Geometry: final body of the model. Coordinates: model frame, mm. Face numbers are marked on the shaded views. A direction names the side the tool comes from. Round coordinates to 2 decimals unless told otherwise and drop trailing zeros. Order: outer loops, then holes, each group sorted by start corner. A loop starts at its lowest first (then second) coordinate and runs counter-clockwise, first axis right, second up. Notation, with made-up numbers: (57, 13) -> (87, 13) arc R24 ccw to (87, 41) -> close; hole circle Ø7 at (23, -29). An arc over 180 degrees is marked (long way). Put each result on its own line as item: value.
```python
from build123d import *

# Parameters (mm, degrees)
SKETCH1_W           = 128.5875
SKETCH1_H           = 144.4625
BOSS_EXTRUDE1_DEPTH = 61.07176
SHELL1_T            = 6.35
SKETCH2_R           = 8.73125
SKETCH2_R_2         = 19.84375
SKETCH2_W           = 45.72
SKETCH2_H           = 63.1825
SKETCH2_W_2         = 69.215
SKETCH2_H_2         = 23.8125
CUT_EXTRUDE1_DEPTH  = 126.344509202
SKETCH3_W           = 31.75
SKETCH3_H           = 66.675
CUT_EXTRUDE2_DEPTH  = 6.35
SKETCH4_R           = 19.84375
SKETCH4_R_2         = 16.66875
BOSS_EXTRUDE2_DEPTH = 1.5875
SKETCH5_W           = 63.5
SKETCH5_H           = 12.7
CUT_EXTRUDE3_DEPTH  = 6.35
FILLET1_R           = 9.525
FILLET2_R           = 3.175


with BuildPart() as part:
    # Sketch1 → Boss-Extrude1 (new body)
    with BuildSketch(Plane.XY):
        Rectangle(SKETCH1_W, SKETCH1_H)
    extrude(amount=-BOSS_EXTRUDE1_DEPTH)

    # Shell1
    shell1_openings = [part.faces().sort_by_distance(p)[0] for p in [
        (0, 0, -61.07176),
    ]]
    offset(amount=SHELL1_T, openings=shell1_openings, kind=Kind.INTERSECTION)

    # Sketch2 → Cut-Extrude1 (cut, through all)
    with BuildSketch(Plane.XY.offset(6.35)):
        with Locations((-31.75, 50.8)):
            Circle(SKETCH2_R)
        with Locations((-31.75, 9.525)):
            Circle(SKETCH2_R_2)
        with Locations((26.19375, 25.4)):
            Rectangle(SKETCH2_W, SKETCH2_H)
        with Locations((11.90625, -41.275)):
            Rectangle(SKETCH2_W_2, SKETCH2_H_2)
    extrude(amount=-CUT_EXTRUDE1_DEPTH, mode=Mode.SUBTRACT)

    # Sketch3 → Cut-Extrude2 (cut)
    with BuildSketch(Plane(origin=(70.64375, 0, 0), x_dir=(0, 0, -1), z_dir=(1, 0, 0))):
        with Locations((31.39694, -13.43025)):
            Rectangle(SKETCH3_W, SKETCH3_H)
    extrude(amount=-CUT_EXTRUDE2_DEPTH, mode=Mode.SUBTRACT)

    # Sketch4 → Boss-Extrude2 (add)
    with BuildSketch(Plane.XY.offset(6.35)):
        with Locations((-31.75, 9.525)):
            Circle(SKETCH4_R)
        with Locations((-31.75, 9.525)):
            Circle(SKETCH4_R_2, mode=Mode.SUBTRACT)
    extrude(amount=-BOSS_EXTRUDE2_DEPTH)

    # Sketch5 → Cut-Extrude3 (cut)
    with BuildSketch(Plane(origin=(0, 78.58125, 0), x_dir=(1, 0, 0), z_dir=(0, 1, 0))):
        with Locations((0, 54.72176)):
            Rectangle(SKETCH5_W, SKETCH5_H)
    extrude(amount=-CUT_EXTRUDE3_DEPTH, mode=Mode.SUBTRACT)

    # Fillet1
    fillet1_edges = [part.edges().sort_by_distance(p)[0] for p in [
        (0, -78.58125, 6.35),
        (70.64375, 0, 6.35),
        (0, 78.58125, 6.35),
        (-70.64375, 0, 6.35),
        (-70.64375, -78.58125, -27.36088),
        (70.64375, -78.58125, -27.36088),
        (70.64375, 78.58125, -27.36088),
        (-70.64375, 78.58125, -27.36088),
    ]]
    fillet(fillet1_edges, radius=FILLET1_R)

    # Fillet2
    fillet2_edges = [part.edges().sort_by_distance(p)[0] for p in [
        (-64.29375, 0, 0),
        (-64.29375, -72.23125, -30.53588),
        (0, 72.23125, 0),
        (-64.29375, 72.23125, -30.53588),
        (64.29375, 72.23125, -30.53588),
        (64.29375, -72.23125, -30.53588),
        (0, -72.23125, 0),
        (64.29375, 0, 0),
    ]]
    fillet(fillet2_edges, radius=FILLET2_R)


solid = part.part
```
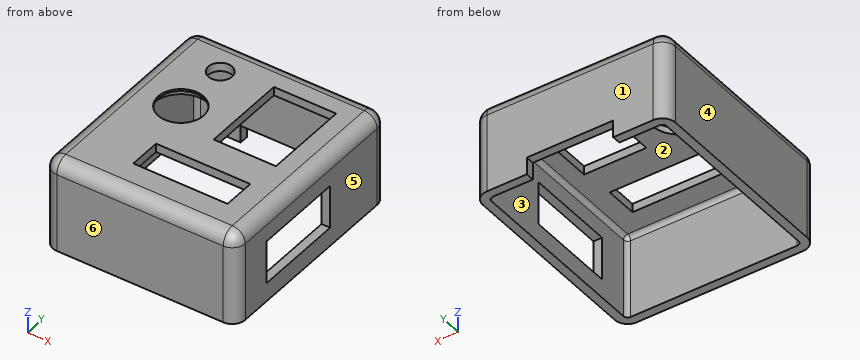
1. Draft query along X for the marked faces 3, 4, 5 and 6. Return one class per face: +X half, -X half, draft (parallel to the pull), parting line (faces both ways), or undercut.
Ans:
face 3: undercut
face 4: -X half
face 5: +X half
face 6: draft
2. Contact query for flat-ended pins moving along their axis: P1, Ø7, axis at x = 29, z = 4, coming from the +Y side; P2, Ø1.9, axis at y = 75, z = -55, coming from the -X side; P3, Ø5, axis at y = -46, z = 3.5, coming from the -X side. Output: stop coordinate, or through.
Ans:
P1: y = 77.84
P2: x = -69.23
P3: x = -69.68
3. Cut plane B-B on x = 53. Return loops of the section in (y, z) (3 decimals), and give its area (3 significant figures).
Ans:
outline: (-78.581, -61.072) -> (-72.231, -61.072) -> (-72.231, -3.175) arc R3.175 cw to (-69.056, 0) -> (69.056, 0) arc R3.175 cw to (72.231, -3.175) -> (72.231, -61.072) -> (78.581, -61.072) -> (78.581, -3.175) arc R9.525 ccw to (69.056, 6.35) -> (-69.056, 6.35) arc R9.525 ccw to (-78.581, -3.175) -> close
area: 1,740 mm²
4. Material intervals for probe 1 along Y at (x, z) = (48.5, -3); probe 2 along X at (y, z) = (19, -53.5); probe 3 along Z at (x, y) = (-0.5, 53), sorted ascending.
Ans:
probe 1: -78.58 to -72.23, 72.23 to 78.58
probe 2: -70.64 to -64.29, 64.29 to 70.64
probe 3: 0 to 6.35
5. Set-up query: the marked faces 1 and 2. Return all of +Z, -Z, +X, -X, +Y, -Y with unobstructed straight access to the full face (end or side cutting, diameter ignored); none if empty.
Ans:
face 1: +Z, -Z, +X, -X, +Y
face 2: -Z
6. Cut plane D-D on z = -21. Return loops of the section in (x, y) (3 decimals).
Ans:
outline: (-70.644, -69.056) arc R9.525 ccw to (-61.119, -78.581) -> (61.119, -78.581) arc R9.525 ccw to (70.644, -69.056) -> (70.644, -46.768) -> (64.294, -46.768) -> (64.294, -69.056) arc R3.175 cw to (61.119, -72.231) -> (-61.119, -72.231) arc R3.175 cw to (-64.294, -69.056) -> (-64.294, 69.056) arc R3.175 cw to (-61.119, 72.231) -> (61.119, 72.231) arc R3.175 cw to (64.294, 69.056) -> (64.294, 19.907) -> (70.644, 19.907) -> (70.644, 69.056) arc R9.525 ccw to (61.119, 78.581) -> (-61.119, 78.581) arc R9.525 ccw to (-70.644, 69.056) -> close
7. Cut plane C-C on z = -12.5. Return loops of the section in (x, y) (3 decimals).
Ans:
outline: (-70.644, -69.056) arc R9.525 ccw to (-61.119, -78.581) -> (61.119, -78.581) arc R9.525 ccw to (70.644, -69.056) -> (70.644, 69.056) arc R9.525 ccw to (61.119, 78.581) -> (-61.119, 78.581) arc R9.525 ccw to (-70.644, 69.056) -> close; hole (-64.294, -69.056) arc R3.175 ccw to (-61.119, -72.231) -> (61.119, -72.231) arc R3.175 ccw to (64.294, -69.056) -> (64.294, 69.056) arc R3.175 ccw to (61.119, 72.231) -> (-61.119, 72.231) arc R3.175 ccw to (-64.294, 69.056) -> close
8. Cut plane A-A on y = -37.5. Return loops of the section in (x, z) (3 decimals), and give its area (3 significant figures).
Ans:
outline: (-70.644, -61.072) -> (-64.294, -61.072) -> (-64.294, -3.175) arc R3.175 cw to (-61.119, 0) -> (-22.701, 0) -> (-22.701, 6.35) -> (-61.119, 6.35) arc R9.525 ccw to (-70.644, -3.175) -> close; (46.514, 0) -> (61.119, 0) arc R3.175 cw to (64.294, -3.175) -> (64.294, -15.522) -> (70.644, -15.522) -> (70.644, -3.175) arc R9.525 ccw to (61.119, 6.35) -> (46.514, 6.35) -> close; (64.294, -61.072) -> (70.644, -61.072) -> (70.644, -47.272) -> (64.294, -47.272) -> close
area: 997 mm²
